from build123d import *

# Parameters (mm, degrees)
F0_R     = 0.396875
F0_W     = 2.54
F0_H     = 55.765484
F1_DEPTH = 3.175


with BuildPart() as f1:
    # F0 (on Top) → F1 (new body)
    with BuildSketch(Plane.XY):
        Polygon((-12.7, 11.43), (-22.225, 11.43), (-22.225, 8.255), (-20.955, 8.255), (-20.955, 10.16), (-14.605, 10.16), (-14.605, 0), (-20.955, 0), (-20.955, 1.905), (-22.225, 1.905), (-22.225, -1.27), (-12.7, -1.27), (-12.7, 1.27), align=None)
        with Locations((-21.59, 1.397)):
            Circle(F0_R, mode=Mode.SUBTRACT)
        with Locations((-21.59, 8.763)):
            Circle(F0_R, mode=Mode.SUBTRACT)
        Polygon((12.7, 1.27), (-12.7, 1.27), (-12.7, -1.27), (-11.409179, -1.27), (-1.27, -1.27), (1.27, -1.27), (11.409179, -1.27), (12.7, -1.27), align=None)
        Polygon((12.7, 11.43), (12.7, 1.27), (12.7, -1.27), (22.225, -1.27), (22.225, 1.905), (20.955, 1.905), (20.955, 0), (14.605, 0), (14.605, 10.16), (20.955, 10.16), (20.955, 8.255), (22.225, 8.255), (22.225, 11.43), align=None)
        with Locations((21.59, 1.397)):
            Circle(F0_R, mode=Mode.SUBTRACT)
        with Locations((21.59, 8.763)):
            Circle(F0_R, mode=Mode.SUBTRACT)
        with BuildLine():
            Line((-11.409179, -1.27), (-12.7, -1.27))
            Line((-12.7, -1.27), (-0.624757, -67.683834))
            ThreePointArc((-0.624757, -67.683834), (0, -68.205242), (0.624757, -67.683834))
            Line((0.624757, -67.683834), (12.7, -1.27))
            Line((12.7, -1.27), (11.409179, -1.27))
            Line((11.409179, -1.27), (1.27, -57.035484))
            Line((1.27, -57.035484), (0.008035, -63.976291))
            ThreePointArc((0.008035, -63.976291), (0.5641, -64.211582), (0.79375, -64.77))
            ThreePointArc((0.79375, -64.77), (-0.558418, -65.3341), (-0.008035, -63.976291))
            Line((-0.008035, -63.976291), (-1.27, -57.035484))
            Line((-1.27, -57.035484), (-11.409179, -1.27))
        make_face()
        with Locations((0, -29.152742)):
            Rectangle(F0_W, F0_H)
        with BuildLine():
            Line((1.27, -57.035484), (-1.27, -57.035484))
            Line((-1.27, -57.035484), (-0.008035, -63.976291))
            ThreePointArc((-0.008035, -63.976291), (0, -63.97625), (0.008035, -63.976291))
            Line((0.008035, -63.976291), (1.27, -57.035484))
        make_face()
    extrude(amount=F1_DEPTH)


solid = f1.part
Verification items for the finished model (mm, model axes). A direction names the side the tool comes from. Round coordinates to 2 decimals unless told otherwise and drop trailing zeros. Order: outer loops, then holes, each group sorted by start corner. A loop starts at its lowest first (then second) coordinate and runs counter-clockwise, first axis right, second up.
1. Release check for a two-part mould opening along Y. For faces 1 (the flat face through (6.41, -28.76, 1.57)), 2 (the flat face through (18, 11.43, 2)), 3 (the flat face through (6.58, -34.94, 1.57)) record: +Y half, -Y half, draft (parallel to the pull), parting line (faces both ways), or undercut.
Final values:
face 1: undercut
face 2: +Y half
face 3: -Y half
2. Section check B-B on y = -49.5. Record the cut outline in (x, z) (3 decimals), then the cut area to 3 significant figures.
Final values:
outline: (-3.931, 0) - (-2.64, 0) - (-2.64, 3.175) - (-3.931, 3.175) - close; (-1.27, 0) - (1.27, 0) - (1.27, 3.175) - (-1.27, 3.175) - close; (2.64, 0) - (3.931, 0) - (3.931, 3.175) - (2.64, 3.175) - close
area: 16.3 mm2
3. Section check A-A on x = -17. Record the cut outline in (y, z) (3 decimals).
Final values:
outline: (-1.27, 0) - (0, 0) - (0, 3.175) - (-1.27, 3.175) - close; (10.16, 0) - (11.43, 0) - (11.43, 3.175) - (10.16, 3.175) - close
4. Access from +Z, -Z, +X, -X, +Y, -Y to the whole of each face (thin tool, end or side, straight path). Record for faces 4 (the flat face through (0, 1.27, 2)), 5 (the flat face through (-1.27, -30, 2)), 6 (the flat face through (17, -1.27, 2)), 7 (the flat face through (22.225, 0, 2)), 8 (the flat face through (0, -25, 0)).
Final values:
face 4: +Z, -Z, +Y
face 5: +Z, -Z
face 6: +Z, -Z, +X, -Y
face 7: +Z, -Z, +X, +Y, -Y
face 8: -Z, +X, -X, +Y, -Y
5. Thickness scan on L1, parallel to X at y = -37, z = 3.05; L2, parallel to X at y = -24, z = 0.3; L3, parallel to Y at x = -14, z = 2.7. Record the ranges inside material, lowest first.
Final values:
L1: x = -6.2 to -4.91, -1.27 to 1.27, 4.91 to 6.2
L2: x = -8.57 to -7.28, -1.27 to 1.27, 7.28 to 8.57
L3: y = -1.27 to 11.43
6. Go/stop test with flat-tipped pins: P1, Ø1, axis at y = 4.5, z = 1.5, coming from the +X side (3 decimals); P2, Ø1, axis at x = 21.5, z = 2, coming from the -Y side; P3, Ø1, axis at x = -5.5, z = 1, coming from the +Y side; P4, Ø1, axis at x = 12, y = -12, coming from the -Z side. Record where each tip stops, or that it passes through.
Final values:
P1: stops at x = 14.605
P2: stops at y = -1.27
P3: stops at y = 1.27
P4: passes through
7. Section check D-D on z = 0.85. State how many separate pieces and enclosed holes the cut face has, then the cut area to 3 significant figures.
Final values:
separate pieces: 1
enclosed holes: 7
area: 477 mm2
8. Section check C-C on x = -4. Record the cut outline in (y, z) (3 decimals).
Final values:
outline: (-49.12, 0) - (-42.02, 0) - (-42.02, 3.175) - (-49.12, 3.175) - close; (-1.27, 0) - (1.27, 0) - (1.27, 3.175) - (-1.27, 3.175) - close
